```python
from build123d import *

# Parameters (mm, degrees)
F1_DEPTH = 25
F2_DEPTH = 1
F3_W     = 108.879238
F3_H     = 87.930533
F4_DEPTH = 24


with BuildPart() as f1:
    # F0 (on Front) → F1 (new body)
    with BuildSketch(Plane.XZ):
        Polygon((-45.439619, 45), (-50.439619, 45), (-45.489871, 40.050253), (45.489871, 40.050253), (50.439619, 45), (3.5, 45), (-3.5, 45), align=None)
        Polygon((-55.439619, 45), (-55.439619, 40), (-50.489871, 35.050253), (-50.489871, -35.050253), (-55.439619, -40), (-55.439619, -44.930533), (-50.439619, -44.930533), (-45.489871, -40.050253), (45.489871, -40.050253), (50.370151, -44.930533), (50.439619, -44.930533), (55.439619, -44.930533), (55.439619, -40), (50.489871, -35.050253), (50.489871, 35.050253), (55.439619, 40), (55.439619, 45), (50.439619, 45), (45.489871, 40.050253), (-45.489871, 40.050253), (-50.439619, 45), align=None)
        Polygon((55.439619, 3.5), (55.439619, 40), (50.489871, 35.050253), (50.489871, -35.050253), (55.439619, -40), (55.439619, -39.930533), (55.439619, -3.5), align=None)
        Polygon((-45.489871, -40.050253), (-50.439619, -44.930533), (-3.5, -44.930533), (3.5, -44.930533), (50.370151, -44.930533), (45.489871, -40.050253), align=None)
        Polygon((-55.439619, 40), (-55.439619, 3.5), (-55.439619, -3.5), (-55.439619, -39.930533), (-55.439619, -40), (-50.489871, -35.050253), (-50.489871, 35.050253), align=None)
    extrude(amount=-F1_DEPTH)

    # F0 (on Front) → F2 (cut)
    with BuildSketch(Plane.XZ):
        Polygon((-55.439619, 45), (-55.439619, 40), (-50.489871, 35.050253), (-50.489871, -35.050253), (-55.439619, -40), (-55.439619, -44.930533), (-50.439619, -44.930533), (-45.489871, -40.050253), (45.489871, -40.050253), (50.370151, -44.930533), (50.439619, -44.930533), (55.439619, -44.930533), (55.439619, -40), (50.489871, -35.050253), (50.489871, 35.050253), (55.439619, 40), (55.439619, 45), (50.439619, 45), (45.489871, 40.050253), (-45.489871, 40.050253), (-50.439619, 45), align=None)
    extrude(amount=-F2_DEPTH, mode=Mode.SUBTRACT)

    # F3 (on face) → F4 (cut)
    with BuildSketch(Plane(origin=(0, 25, 0), x_dir=(-1, 0, 0), z_dir=(0, 1, 0))):
        with Locations((0, 0.034734)):
            Rectangle(F3_W, F3_H)
    extrude(amount=-F4_DEPTH, mode=Mode.SUBTRACT)


solid = f1.part
```
Source: CAD feature listing. Evaluate the final solid. Frame: model axes, mm. A direction names the side the tool comes from. Round coordinates to 2 decimals unless told otherwise and drop trailing zeros. Order: outer loops, then holes, each group sorted by start corner. A loop starts at its lowest first (then second) coordinate and runs counter-clockwise, first axis right, second up. Notation, with made-up numbers: (-16, 27) -> (5, 27) arc R25 ccw to (5, 58) -> close; hole circle Ø9 at (-33, -1). An arc over 180 degrees is marked (long way). One line per item, written item: value. Start each with the question number.
Q1. Material intervals for probe 1 along Z at (x, y) = (28.5, 22.5); probe 2 along X at (y, z) = (20.75, 40); probe 3 along Y at (x, z) = (45, 41), sorted ascending.
Q2. Section query B-B (z = -29). Return the cut outline in (x, y), plus the area to 3 significant figures.
Q3. Section query A-A (x = -8). Return the cut outline in (y, z), plus the area to 3 significant figures.
Q4. Access query for faces 1 (the flat face through (48, 0.49, 42.56)), 2 (the flat face through (-54.44, 13, -1)), 3 (the flat face through (-47.93, 0.49, 42.49)), 4 (the flat face through (52.93, 0.49, 37.49)), 5 (the flat face through (-52.93, 0.49, -37.49)). Directions: +Z, -Z, +X, -X, +Y, -Y. A direction counts if a zero-diameter tool reaches every point of the face in a straight line with its end or side. Return the directions, or none.
Q5. Section query C-C (y = 6). Return the cut outline in (x, z), plus the area to 3 significant figures.
Q6. Draft query along X for faces 6 (the flat face through (-1, 0, -42)), 7 (the flat face through (55.44, 12, -1)), 8 (the flat face through (1, 13, -43.931)). Return one class per face: pulls with the +X half, pulls with the -X half, needs draft (parallel to the pull), parting line crosses it, or undercut.
Q7. Pin query (flat end, axial travel): pin 1 (6.5 mm diameter, centred on x = 52.5, z = 42, fed in from -Y); pin 2 (1.2 mm diameter, centred on x = 24.5, z = -42, fed in from +Y). Return the tip coordinate at first contact, or that it passes through.
Findings below:
1. probe 1: -44.93 to -43.93, 44 to 45
1. probe 2: -55.44 to -54.44, 54.44 to 55.44
1. probe 3: 0 to 1
2. outline: (-55.44, 0) -> (-50.49, 0) -> (-50.49, 1) -> (-54.44, 1) -> (-54.44, 25) -> (-55.44, 25) -> close; (50.49, 0) -> (55.44, 0) -> (55.44, 25) -> (54.44, 25) -> (54.44, 1) -> (50.49, 1) -> close
2. area: 57.9 mm²
3. outline: (0, -44.93) -> (25, -44.93) -> (25, -43.93) -> (1, -43.93) -> (1, -40.05) -> (0, -40.05) -> close; (0, 40.05) -> (1, 40.05) -> (1, 44) -> (25, 44) -> (25, 45) -> (0, 45) -> close
3. area: 57.8 mm²
4. face 1: +X, -Y
4. face 2: +Y
4. face 3: -X, -Y
4. face 4: +Z, -Y
4. face 5: -Z, -Y
5. outline: (-55.44, -44.93) -> (55.44, -44.93) -> (55.44, 45) -> (-55.44, 45) -> close; hole (-54.44, -43.93) -> (54.44, -43.93) -> (54.44, 44) -> (-54.44, 44) -> close
5. area: 398 mm²
6. face 6: needs draft
6. face 7: pulls with the +X half
6. face 8: undercut
7. pin 1: y = 1
7. pin 2: y = 1
